Part model, mm, in its own coordinate system. Give positions to 0.01 mm unless a question says otherwise; leave off trailing zeros. Order: outer loops, then holes, each group sorted by start corner. A loop starts at its lowest first (then second) coordinate and runs counter-clockwise, first axis right, second up. Notation, with made-up numbers: M 39.25,46.25 L 47.25,46.25 A19 cw 47.25,50.25 Z; hole C 32.25,26 d8. An arc over 180 degrees is marked long. Answer as a JSON object with one key per item and string values.
Autodesk Inventor part; units mm, degrees
ref_plane "YZ Plane" through (0, 0, 0) normal (1, 0, 0) x (0, 1, 0)
ref_plane "XZ Plane" through (0, 0, 0) normal (0, 1, 0) x (-1, 0, 0)
ref_plane "XY Plane" through (0, 0, 0) normal (0, 0, 1) x (1, 0, 0)
sketch "Sketch1" plane through (0, 0, 0) normal (1, 0, 0) x (0, 1, 0)
  line L0 (0, 0) -> (81, 0)
  line L1 (81, 0) -> (81, -50)
  line L2 (81, -50) -> (0, -50)
  line L3 (0, -50) -> (0, 0)
  circle A0 centre (71, -15) radius 2
  circle A1 centre (71, -34) radius 2
  circle A2 centre (14, -15) radius 2
  circle A3 centre (14, -34) radius 2
  dimension "d0" = 81
  dimension "d1" = 50
  dimension "d2" = 4
  dimension "d3" = 15
  dimension "d4" = 4
  dimension "d5" = 16
  dimension "d6" = 4
  dimension "d7" = 15
  dimension "d8" = 4
  dimension "d9" = 57
  dimension "d11" = 10
  dimension "d12" = 57
  dimension "d13" = 10
extrude "Extrusion1" add sketch "Sketch1" along normal blind 3
sketch "Sketch5" plane through (0, 81, 0) normal (0, 1, 0) x (1, 0, 0)
  circle A0 centre (7, 25) radius 4
  line L0 (0, 0) -> (3, 0)
  line L1 (3, 50) -> (3, 0)
  dimension "d26" = 8
  dimension "d27" = 25
  dimension "d28" = 4
extrude "Extrusion3" add sketch "Sketch5" against normal blind 81
sketch "Sketch8" plane through (0, 81, 0) normal (0, 1, 0) x (1, 0, 0)
  circle A0 centre (7, 25) radius 4
  line L0 (0, 0) -> (3, 0)
  line L1 (3, 50) -> (3, 25)
  point P0 (3, 29)
  dimension "d33" = 8
  dimension "d34" = 25
  dimension "d35" = 4
extrude "Extrusion5" cut sketch "Sketch8" against normal blind 81
1. Two-plate mould, pull along Y, no slides. Class faces 1 (the flat face through (1, 0, -25)), 2 (the cylindrical face through (1, 14, -17)), 3 (the flat face through (1, 41, -50)), 4 (the flat face through (1, 81, -25)): +Y half, -Y half, draft (parallel to the pull), parting line (faces both ways), or undercut.
Worked answers:
{"face 1": "-Y half", "face 2": "undercut", "face 3": "draft", "face 4": "+Y half"}
2. Cut at A-A on y = 71. Give the cut face in (x, z), plus the area to 3 significant figures.
Worked answers:
{"outline": "M 0,-50 L 3,-50 L 3,-36 L 0,-36 Z; M 0,-32 L 3,-32 L 3,-17 L 0,-17 Z; M 0,-13 L 3,-13 L 3,0 L 0,0 Z", "area": "126 mm^2"}
3. Cut at B-B on z = -34. Give the cut face in (x, y), plus the area to 3 significant figures.
Worked answers:
{"outline": "M 0,0 L 3,0 L 3,12 L 0,12 Z; M 0,16 L 3,16 L 3,69 L 0,69 Z; M 0,73 L 3,73 L 3,81 L 0,81 Z", "area": "219 mm^2"}
4. Pin check, flat tip, straight feed: P1, Ø4.5, axis at y = 14, z = -34, coming from the +X side. Stop position of the tip, or through.
Worked answers:
{"P1": "stops at x = 3"}
5. Probe line 1 along Z through (x, y) = (1.3, 71); line 2 along Y through (x, z) = (2.5, -13.5). List the from-to ranges inside material, lowest first.
Worked answers:
{"line 1": "z = -50 to -36, -32 to -17, -13 to 0", "line 2": "y = 0 to 12.68, 15.32 to 69.68, 72.32 to 81"}
